Here's how the part is built. I have some questions about the finished solid (model axes, mm). Face numbers are marked on the shaded views. Round coordinates to 2 decimals unless told otherwise and drop trailing zeros. Order: outer loops, then holes, each group sorted by start corner. A loop starts at its lowest first (then second) coordinate and runs counter-clockwise, first axis right, second up.
```python
from build123d import *

# Parameters (mm, degrees)
SKETCH_1_R      = 4
SKETCH_1_R_2    = 2
EXTRUDE_1_DEPTH = 5


with BuildPart() as part:
    # 草图1 → 凸台-拉伸1 (new body)
    with BuildSketch(Plane(origin=(0, 0, 0), x_dir=(1, 0, 0), z_dir=(0, 1, 0))):
        Polygon((-34.5, 21.15), (34.5, 21.15), (34.5, 16.15), (39.5, 16.15), (39.5, 6.15), (34.5, 6.15), (34.5, -6.15), (39.5, -6.15), (39.5, -16.15), (34.5, -16.15), (34.5, -21.15), (24.5, -21.15), (24.5, -26.15), (14.5, -26.15), (14.5, -21.15), (-14.5, -21.15), (-14.5, -26.15), (-24.5, -26.15), (-24.5, -21.15), (-34.5, -21.15), (-34.5, -16.15), (-39.5, -16.15), (-39.5, -6.15), (-34.5, -6.15), (-34.5, 6.15), (-39.5, 6.15), (-39.5, 16.15), (-34.5, 16.15), align=None)
        with Locations(Location((10.5, 0, 0), (0, 0, 270))):
            Circle(SKETCH_1_R, mode=Mode.SUBTRACT)
        with Locations(Location((-21.5, 0, 0), (0, 0, 270))):
            Circle(SKETCH_1_R, mode=Mode.SUBTRACT)
        with Locations(Location((-7.5, 0, 0), (0, 0, 270))):
            Circle(SKETCH_1_R_2, mode=Mode.SUBTRACT)
        with Locations(Location((28.5, 0, 0), (0, 0, 270))):
            Circle(SKETCH_1_R_2, mode=Mode.SUBTRACT)
    extrude(amount=EXTRUDE_1_DEPTH)


solid = part.part
```
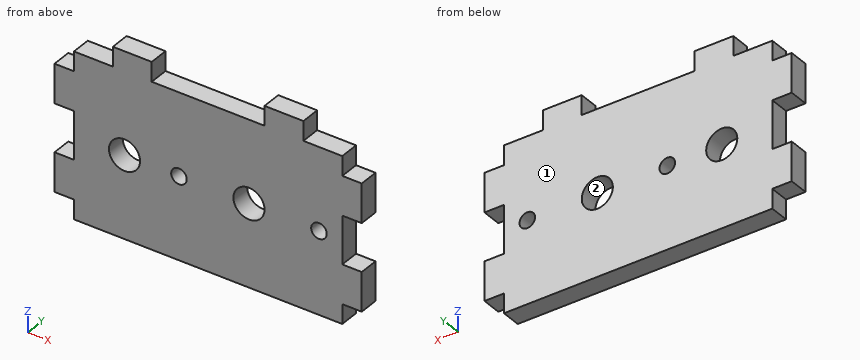
1. I'm going to push flat-ended pins straight in: P1, Ø2.5, axis at x = -28.5, y = 3.5, coming from the +Z side; P2, Ø1.5, axis at y = 2, z = 18, coming from the -X side; P3, Ø2.5, axis at x = -36, y = 3.5, coming from the -Z side. Where does each tip first touch, or does it pass through?
Evaluation:
P1: stops at z = 21.15
P2: stops at x = -34.5
P3: stops at z = -16.15
2. If we section it at B-B, the plane x = 10.5: Write out the boundary of the cut face in (y, z), and give its area (4 significant figures).
Evaluation:
outline: (0, -21.15) - (5, -21.15) - (5, -4) - (0, -4) - close; (0, 4) - (5, 4) - (5, 21.15) - (0, 21.15) - close
area: 171.5 mm2
3. If we section it at C-C, the plane y = 4.15: State how many separate pieces and enclosed holes the cut face has, and give its area (3 significant figures).
Evaluation:
separate pieces: 1
enclosed holes: 4
area: 3,090 mm2
4. If we mould it in two halves opening along Z, with no side actions, what happens to the marked faces 1 and 2? For each: released by +Z, released by -Z, zero draft, split by the parting line, or undercut.
Evaluation:
face 1: zero draft
face 2: undercut
5. If we section it at A-A, the plane z = 0: Write out the boundary of the cut face in (x, y).
Evaluation:
outline: (-34.5, 0) - (-25.5, 0) - (-25.5, 5) - (-34.5, 5) - close; (-17.5, 0) - (-9.5, 0) - (-9.5, 5) - (-17.5, 5) - close; (-5.5, 0) - (6.5, 0) - (6.5, 5) - (-5.5, 5) - close; (14.5, 0) - (26.5, 0) - (26.5, 5) - (14.5, 5) - close; (30.5, 0) - (34.5, 0) - (34.5, 5) - (30.5, 5) - close
6. If we section it at D-D, the plane x = 28.5: Write out the boundary of the cut face in (y, z), and give its area (4 significant figures).
Evaluation:
outline: (0, -21.15) - (5, -21.15) - (5, -2) - (0, -2) - close; (0, 2) - (5, 2) - (5, 21.15) - (0, 21.15) - close
area: 191.5 mm2
7. I need wall thicknesses on probe 1 along X at (y, z) = (1.9, 0); probe 2 along X at (y, z) = (1, 3.5); probe 3 along X at (y, z) = (3.75, 22). Which ranges of each line are inside material? Lowest first, please.
Evaluation:
probe 1: x = -34.5 to -25.5, -17.5 to -9.5, -5.5 to 6.5, 14.5 to 26.5, 30.5 to 34.5
probe 2: x = -34.5 to -23.44, -19.56 to 8.56, 12.44 to 34.5
probe 3: x = -24.5 to -14.5, 14.5 to 24.5
